from build123d import *

# Parameters (mm, degrees)
SKETCH1_W           = 30
SKETCH1_H           = 52.4
BOSS_EXTRUDE1_DEPTH = 10
CUT_EXTRUDE1_DEPTH  = 30
SKETCH3_R           = 1.55
CUT_EXTRUDE2_DEPTH  = 14
CUT_EXTRUDE3_START  = -4
SKETCH3_4_R         = 3
SKETCH3_4_R_2       = 1.55
CUT_EXTRUDE3_DEPTH  = 12
CUT_EXTRUDE4_START  = -1.5
SKETCH3_7_R         = 3
SKETCH3_7_R_2       = 1.55
CUT_EXTRUDE4_DEPTH  = 60.702614474


with BuildPart() as part:
    # Sketch1 → Boss-Extrude1 (new body)
    with BuildSketch(Plane(origin=(0, 0, 0), x_dir=(1, 0, 0), z_dir=(0, 1, 0))):
        with Locations((15, 26.2)):
            Rectangle(SKETCH1_W, SKETCH1_H)
    extrude(amount=BOSS_EXTRUDE1_DEPTH)

    # Sketch2 → Cut-Extrude1 (cut)
    with BuildSketch(Plane(origin=(30, 0, 0), x_dir=(0, 0, -1), z_dir=(1, 0, 0))):
        with BuildLine():
            Line((52.4, 10), (0, 10))
            Line((0, 10), (0, 0))
            add(Edge.make_bspline(
                [(52.4, 10), (26.797572393, 1.464832173), (0, 0)],
                knots=[0, 0, 0, 1, 1, 1], degree=2))
        make_face()
    extrude(amount=-CUT_EXTRUDE1_DEPTH, mode=Mode.SUBTRACT)

    # Sketch3 → Cut-Extrude2 (cut)
    with BuildSketch(Plane(origin=(0, 0, 0), x_dir=(-1, 0, 0), z_dir=(0, -1, 0))):
        with Locations(Location((-15, 35.33, 0), (0, 0, 90))):
            Circle(SKETCH3_R)
        with Locations(Location((-15, 17.65, 0), (0, 0, 90))):
            Circle(SKETCH3_R)
    extrude(amount=-CUT_EXTRUDE2_DEPTH, mode=Mode.SUBTRACT)

    # Sketch3_4 → Cut-Extrude3 (cut)
    with BuildSketch(Plane(origin=(0, 0, 0), x_dir=(-1, 0, 0), z_dir=(0, -1, 0)).offset(CUT_EXTRUDE3_START)):
        with Locations(Location((-15, 35.33, 0), (0, 0, 90))):
            Circle(SKETCH3_4_R)
        with Locations(Location((-15, 35.33, 0), (0, 0, 90))):
            Circle(SKETCH3_4_R_2, mode=Mode.SUBTRACT)
    extrude(amount=-CUT_EXTRUDE3_DEPTH, mode=Mode.SUBTRACT)

    # Sketch3_7 → Cut-Extrude4 (cut, through all)
    with BuildSketch(Plane(origin=(0, 0, 0), x_dir=(-1, 0, 0), z_dir=(0, -1, 0)).offset(CUT_EXTRUDE4_START)):
        with Locations((-15, 17.65)):
            Circle(SKETCH3_7_R)
        with Locations(Location((-15, 17.65, 0), (0, 0, 90))):
            Circle(SKETCH3_7_R_2, mode=Mode.SUBTRACT)
    extrude(amount=-CUT_EXTRUDE4_DEPTH, mode=Mode.SUBTRACT)


solid = part.part
Read the model definition and answer for the solid it produces. Units are mm, in the model's axes. A direction names the side the tool comes from. Coordinates: 2 decimals unless noted, no trailing zeros. Answer as a JSON object with one key per item and string values.
1) Each of these flat-tipped pins is pushed along its axis until it touches: pin 1 (5 mm diameter, centred on x = 15, z = -35.33, fed in from +Y); pin 2 (4 mm diameter, centred on x = 19.5, z = -43.5, fed in from +Y); pin 3 (5.5 mm diameter, centred on x = 16, z = -18.5, fed in from +Y); pin 4 (6 mm diameter, centred on y = 8, z = -34, fed in from -X). Where does it stop, or does it pass through?
Model answer:
{"pin 1": "stops at y = 4", "pin 2": "stops at y = 7.83", "pin 3": "stops at y = 2.3", "pin 4": "passes through"}
2) A tool of negligible diameter and unlimited length cuts with its end or side. For faces 1 (the face through (14, 4, -37)), 2 (the face through (0, 3, -37)), from which of +Z, -Z, +X, -X, +Y, -Y can it reach the whole face along a straight path? Write none if from no direction.
Model answer:
{"face 1": "+Y", "face 2": "+Z, -Z, -X, +Y, -Y"}
3) Consider line 1 along X through (y, z) = (1.45, -35.33); line 2 along X through (y, z) = (4.55, -35.33); line 3 along Y through (x, z) = (13.5, -36). Determine where each line is inside the solid, lowest interval first. Write a range as from..to.
Model answer:
{"line 1": "x = 0..13.45, 16.55..30", "line 2": "x = 0..12, 18..30", "line 3": "y = 0..4"}
